Geometry check sheet. Reference: the model listing, model coordinates, mm. Face numbers are marked on the shaded views. A direction names the side the tool comes from. Round coordinates to 2 decimals unless told otherwise and drop trailing zeros. Write each loop counter-clockwise with the first axis right and the second up, starting at its lowest first coordinate (ties: lowest second). Pieces come first, ordered by that corner, then holes.
Item 1: Draft check along X on the marked faces 3, 4 and 5. Enter one of: pulls with the +X half, pulls with the -X half, needs draft (parallel to the pull), parting line crosses it, or undercut.
Item 2: Cross-section at A-A (y = 4.5). Enter the section's corners in (x, z) (3 decimals), then the cut area to 3 significant figures.
Item 3: Access from +Z, -Z, +X, -X, +Y, -Y to the whole of each face (thin tool, end or side, straight path). Record for the marked faces 1 and 2.
Item 4: Scan lines: probe 1 along Y at (x, z) = (0.5, 2.5); probe 2 along X at (y, z) = (7.25, 0) (3 decimals); probe 3 along Z at (x, y) = (0.25, 2.75). Record each from-to range of solid material in increasing order.
Item 5: Cross-section at B-B (x = 0). Enter the section's corners in (y, z) (3 decimals).
Item 6: Depth check by flat-ended pin: P1, Ø2, axis at y = 5.5, z = 2, coming from the +X side; P2, Ø4, axis at x = 3, y = 1.5, coming from the -Z side; P3, Ø1.5, axis at x = 0.5, y = 3.5, coming from the +Z side (3 decimals). Enter the tip coordinate at first touch or a pass-through.
from build123d import *

# Parameters (mm, degrees)
SKETCH1_R           = 5.5
BOSS_EXTRUDE1_DEPTH = 1
SKETCH2_R           = 5.025
BOSS_EXTRUDE2_DEPTH = 7
CUT_EXTRUDE1_DEPTH  = 7
CHAMFER1_SIZE       = 0.2


with BuildPart() as part:
    # Sketch1 → Boss-Extrude1 (new body)
    with BuildSketch(Plane(origin=(0, 0, 0), x_dir=(1, 0, 0), z_dir=(0, 1, 0))):
        with Locations(Location((0, 0, 0), (0, 0, 270))):
            Circle(SKETCH1_R)
    extrude(amount=BOSS_EXTRUDE1_DEPTH)

    # Sketch2 → Boss-Extrude2 (add)
    with BuildSketch(Plane(origin=(0, 1, 0), x_dir=(1, 0, 0), z_dir=(0, 1, 0))):
        with Locations(Location((0, 0, 0), (0, 0, 270))):
            Circle(SKETCH2_R)
    extrude(amount=BOSS_EXTRUDE2_DEPTH)

    # Sketch3 → Cut-Extrude1 (cut)
    with BuildSketch(Plane.XZ):
        Polygon((3.0022214, 0), (1.5011107, 2.6), (-1.5011107, 2.6), (-3.0022214, 0), (-1.5011107, -2.6), (1.5011107, -2.6), align=None)
    extrude(amount=-CUT_EXTRUDE1_DEPTH, mode=Mode.SUBTRACT)

    # Chamfer1
    chamfer1_edges = [part.edges().sort_by_distance(p)[0] for p in [
        (0, 8, -5.025),
    ]]
    chamfer(chamfer1_edges, length=CHAMFER1_SIZE)


solid = part.part
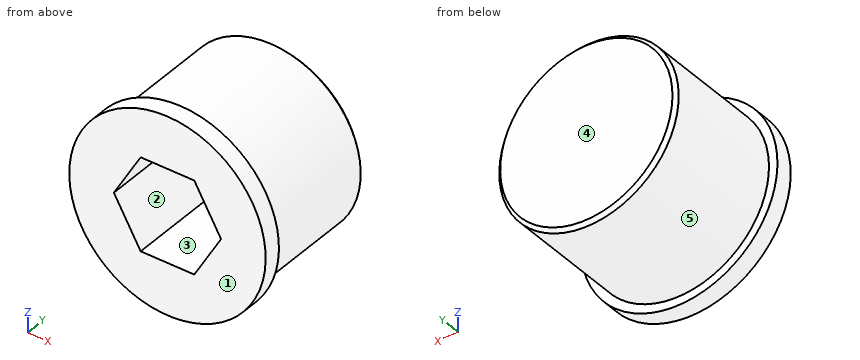
Resolved:
1. face 3: undercut
1. face 4: needs draft
1. face 5: parting line crosses it
2. outline: circle Ø10.05 at (0, 0); hole (-3.002, 0) - (-1.501, -2.6) - (1.501, -2.6) - (3.002, 0) - (1.501, 2.6) - (-1.501, 2.6) - close
2. area: 55.9 mm2
3. face 1: +Z, -Z, +X, -X, -Y
3. face 2: -Y
4. probe 1: y = 7 to 8
4. probe 2: x = -5.025 to 5.025
4. probe 3: z = -5.02 to -2.6, 2.6 to 5.02
5. outline: (0, -5.5) - (1, -5.5) - (1, -5.025) - (7.8, -5.025) - (8, -4.825) - (8, 4.825) - (7.8, 5.025) - (1, 5.025) - (1, 5.5) - (0, 5.5) - (0, 2.6) - (7, 2.6) - (7, -2.6) - (0, -2.6) - close
6. P1: stops at x = 4.92
6. P2: stops at z = -5.4
6. P3: stops at z = 5.025
